from build123d import *

# Parameters (mm, degrees)
SKETCH_1_R          = 10
EXTRUDE_1_DEPTH     = 24
SKETCH_2_R          = 2.6
CUT_EXTRUDE_1_DEPTH = 24


with BuildPart() as part:
    # 草图1 → 凸台-拉伸1 (new body)
    with BuildSketch(Plane(origin=(0, 0, 0), x_dir=(1, 0, 0), z_dir=(0, 1, 0))):
        Polygon((30, 0), (-30, 0), (-30, 10), (-15, 10), (-15, 51), (15, 51), (15, 10), (30, 10), align=None)
        with Locations(Location((0, 31, 0), (0, 0, 270))):
            Circle(SKETCH_1_R, mode=Mode.SUBTRACT)
    extrude(amount=EXTRUDE_1_DEPTH)

    # 草图2 → 切除-拉伸1 (cut)
    with BuildSketch(Plane(origin=(0, 0, -10), x_dir=(-1, 0, 0), z_dir=(0, 0, -1))):
        with Locations((-22.5, 12)):
            Circle(SKETCH_2_R)
        with Locations((22.5, 12)):
            Circle(SKETCH_2_R)
    extrude(amount=-CUT_EXTRUDE_1_DEPTH, mode=Mode.SUBTRACT)


solid = part.part
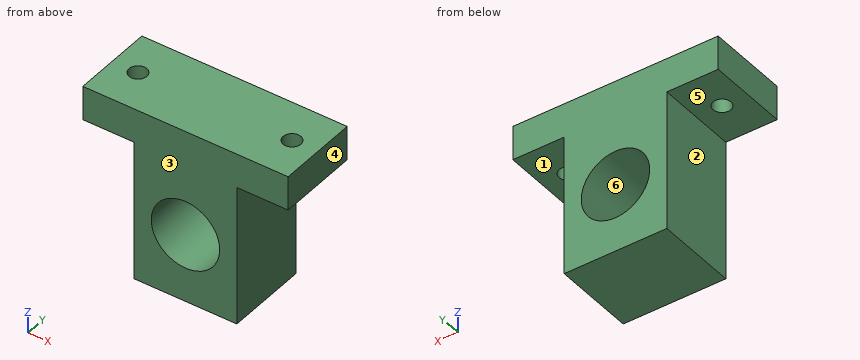
Work out the finished part from the listing and answer in its coordinate system (mm). Face numbers are marked on the shaded views. A direction names the side the tool comes from. Round coordinates to 2 decimals unless told otherwise and drop trailing zeros. Write each loop counter-clockwise with the first axis right and the second up, starting at its lowest first coordinate (ties: lowest second). Pieces come first, ordered by that corner, then holes.
1) A cutting plane is placed at B-B (x = 22.5). Give the vertices of the cut face in (y, z).
2) A cutting plane is placed at A-A (y = 12). Give the vertices of the cut face in (x, z).
3) The mould has two halves that part along Z. Classify the marked faces 4, 5 and 6: pulls with the +Z half, pulls with the -Z half, needs draft (parallel to the pull), parting line crosses it, or undercut.
4) Straight lines are drawn through the part: line 1 (X direction, y = 13.25, z = -31); line 2 (Z direction, x = 21.5, y = 18.5); line 3 (Y direction, x = -22, z = -7). For each, find the intervals that lie inside material, in ascending order.
5) A cutting plane is placed at D-D (y = 3.25). Give the vertices of the cut face in (x, z).
6) Given pin 1 Ø3 at (x, y) = (-24, 17.5) entering from -Z; pin 2 Ø12 at (y, z) = (17, -40.5) entering from -X; pin 3 Ø4.5 at (x, y) = (-22.5, 12) entering from -Z, each flat-ended and moving along its own axis, determine where each tip first touches the part or whether it passes through.
7) A cutting plane is placed at C-C (z = -31). Give the vertices of the cut face in (x, y), plus the area to 3 significant figures.
8) A tool of negligible diameter and unlimited length cuts with its end or side. For the marked faces 1, 2 and 3, from which of +Z, -Z, +X, -X, +Y, -Y can it reach the whole face along a straight path? Write none if from no direction.
Completed:
1. outline: (0, -10) - (9.4, -10) - (9.4, 0) - (0, 0) - close; (14.6, -10) - (24, -10) - (24, 0) - (14.6, 0) - close
2. outline: (-30, -10) - (-25.1, -10) - (-25.1, 0) - (-30, 0) - close; (-19.9, -10) - (-15, -10) - (-15, -51) - (15, -51) - (15, -10) - (19.9, -10) - (19.9, 0) - (-19.9, 0) - close; (25.1, -10) - (30, -10) - (30, 0) - (25.1, 0) - close; hole circle Ø20 at (0, -31)
3. face 4: needs draft
3. face 5: pulls with the -Z half
3. face 6: undercut
4. line 1: x = -15 to -10, 10 to 15
4. line 2: z = -10 to 0
4. line 3: y = 0 to 9.45, 14.55 to 24
5. outline: (-30, -10) - (-15, -10) - (-15, -51) - (15, -51) - (15, -10) - (30, -10) - (30, 0) - (-30, 0) - close; hole circle Ø20 at (0, -31)
6. pin 1: stops at z = -10
6. pin 2: stops at x = -15
6. pin 3: passes through
7. outline: (-15, 0) - (-10, 0) - (-10, 24) - (-15, 24) - close; (10, 0) - (15, 0) - (15, 24) - (10, 24) - close
7. area: 240 mm2
8. face 1: -Z, +X, +Y, -Y
8. face 2: -Z, -X, +Y, -Y
8. face 3: +Z, -Z, +X, -X, -Y
